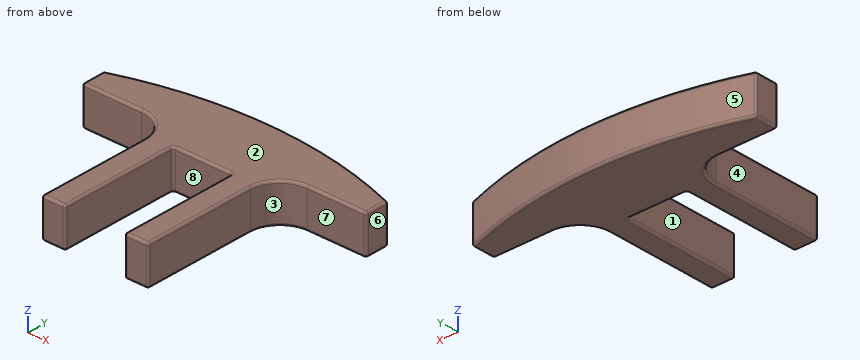
```python
from build123d import *

# Parameters (mm, degrees)
F1_DEPTH = 8.382
F2_R     = 0.508


with BuildPart() as f1:
    # F0 (on Top) → F1 (new body)
    with BuildSketch(Plane.XY):
        with BuildLine():
            Line((-16.819511, 28.70391), (-16.819511, 4.57391))
            Line((-16.819511, 4.57391), (-11.739511, 4.57391))
            Line((-11.739511, 4.57391), (-11.739511, 29.97391))
            Line((-11.739511, 29.97391), (0.960489, 29.97391))
            Line((0.960489, 29.97391), (0.960489, 4.57391))
            Line((0.960489, 4.57391), (6.040489, 4.57391))
            Line((6.040489, 4.57391), (6.040489, 28.70391))
            ThreePointArc((6.040489, 28.70391), (7.900361, 33.194038), (12.390489, 35.05391))
            Line((12.390489, 35.05391), (25.090489, 35.05391))
            Line((25.090489, 35.05391), (25.090489, 40.13391))
            ThreePointArc((25.090489, 40.13391), (-5.389511, 45.511487), (-35.869511, 40.13391))
            Line((-35.869511, 40.13391), (-35.869511, 35.05391))
            Line((-35.869511, 35.05391), (-23.169511, 35.05391))
            ThreePointArc((-23.169511, 35.05391), (-18.679383, 33.194038), (-16.819511, 28.70391))
        make_face()
    extrude(amount=F1_DEPTH)

    # F2
    f2_edges = [f1.edges().sort_by_distance(p)[0] for p in [
        (6.040489, 16.63891, 8.382),
        (3.500489, 4.57391, 8.382),
        (-35.869511, 37.59391, 8.382),
        (-29.519511, 35.05391, 8.382),
        (-18.679383, 33.194038, 8.382),
        (-16.819511, 16.63891, 8.382),
        (-14.279511, 4.57391, 8.382),
        (-11.739511, 17.27391, 8.382),
        (-5.389511, 29.97391, 8.382),
        (0.960489, 17.27391, 8.382),
        (7.900361, 33.194038, 8.382),
        (18.740489, 35.05391, 8.382),
        (25.090489, 37.59391, 8.382),
        (-5.389511, 45.511487, 8.382),
        (-5.389511, 45.511487, 0),
        (25.090489, 37.59391, 0),
        (18.740489, 35.05391, 0),
        (-35.869511, 37.59391, 0),
        (-29.519511, 35.05391, 0),
        (-18.679383, 33.194038, 0),
        (-16.819511, 16.63891, 0),
        (-14.279511, 4.57391, 0),
        (-11.739511, 17.27391, 0),
        (-5.389511, 29.97391, 0),
        (0.960489, 17.27391, 0),
        (3.500489, 4.57391, 0),
        (6.040489, 16.63891, 0),
        (7.900361, 33.194038, 0),
        (25.090489, 40.13391, 4.191),
        (-35.869511, 40.13391, 4.191),
        (12.390489, 35.05391, 4.191),
        (25.090489, 35.05391, 4.191),
        (6.040489, 4.57391, 4.191),
        (6.040489, 28.70391, 4.191),
        (0.960489, 29.97391, 4.191),
        (0.960489, 4.57391, 4.191),
        (-11.739511, 4.57391, 4.191),
        (-11.739511, 29.97391, 4.191),
        (-16.819511, 4.57391, 4.191),
        (-16.819511, 28.70391, 4.191),
        (-35.869511, 35.05391, 4.191),
        (-23.169511, 35.05391, 4.191),
    ]]
    fillet(f2_edges, radius=F2_R)


solid = f1.part
```
Check sheet for the modelled part. Datum: model origin and axes. Units: mm. Face numbers are marked on the shaded views. A direction names the side the tool comes from. Give positions to 0.01 mm unless a question says otherwise; leave off trailing zeros. Write each loop counter-clockwise with the first axis right and the second up, starting at its lowest first coordinate (ties: lowest second). Pieces come first, ordered by that corner, then holes. Notation, with made-up numbers: (10, -19) -> (21, -19) arc R9 cw to (21, -4) -> close; hole circle Ø10 at (76, 75). An arc over 180 degrees is marked (long way). Use CSV: the item, a comma, the result in double quotes. Start each with the question number.
Q1. Depth check by flat-ended pin: P1, Ø2, axis at y = 12.5, z = 2.5, coming from the -X side; P2, Ø2, axis at x = 18.5, z = 5, coming from the -Y side; P3, Ø3, axis at x = -7, z = 7, coming from the -Y side. Enter the tip coordinate at first touch or a pass-through.
Q2. Release check for a two-part mould opening along X. For the marked faces 1, 2 and 3 record: +X half, -X half, draft (parallel to the pull), parting line (faces both ways), or undercut.
Q3. Tool access check on the marked faces 4, 5, 6, 7 and 8. Record the directions out of +Z, -Z, +X, -X, +Y, -Y that give a thin tool (end or side, any length) a straight path to the whole face; none if there is none.
Q4. Scan lines: line 1 along X through (y, z) = (7.5, 4.25); line 2 along X through (y, z) = (10, 8); line 3 along Y through (x, z) = (-12.5, 6.75). Record each from-to range of solid material in increasing order.
Q5. Cross-section at B-B on z = 2.25. Enter the section's corners in (x, y), and give its area (3 significant figures).
Q6. Cross-section at A-A on y = 10. Enter the section's corners in (x, z).
Working result:
1,P1,"stops at x = -16.82"
1,P2,"stops at y = 35.05"
1,P3,"stops at y = 29.97"
2,face 1,"undercut"
2,face 2,"draft"
2,face 3,"+X half"
3,face 4,"+Z, -Z, -X, -Y"
3,face 5,"+Z, -Z, +Y"
3,face 6,"+Z, -Z, +X, +Y, -Y"
3,face 7,"+Z, -Z, +X, -Y"
3,face 8,"+Z, -Z, -Y"
4,line 1,"x = -16.82 to -11.74, 0.96 to 6.04"
4,line 2,"x = -16.8 to -11.76, 0.98 to 6.02"
4,line 3,"y = 4.57 to 45.23"
5,outline,"(-35.87, 35.56) arc R0.51 ccw to (-35.36, 35.05) -> (-23.17, 35.05) arc R6.35 cw to (-16.82, 28.7) -> (-16.82, 5.08) arc R0.51 ccw to (-16.31, 4.57) -> (-12.25, 4.57) arc R0.51 ccw to (-11.74, 5.08) -> (-11.74, 29.47) arc R0.51 cw to (-11.23, 29.97) -> (0.45, 29.97) arc R0.51 cw to (0.96, 29.47) -> (0.96, 5.08) arc R0.51 ccw to (1.47, 4.57) -> (5.53, 4.57) arc R0.51 ccw to (6.04, 5.08) -> (6.04, 28.7) arc R6.35 cw to (12.39, 35.05) -> (24.58, 35.05) arc R0.51 ccw to (25.09, 35.56) -> (25.09, 39.78) arc R0.51 ccw to (24.75, 40.26) arc R89.07 ccw to (-35.53, 40.26) arc R0.51 ccw to (-35.87, 39.78) -> close"
5,area,"921 mm^2"
6,outline,"(-16.82, 0.51) arc R0.51 ccw to (-16.31, 0) -> (-12.25, 0) arc R0.51 ccw to (-11.74, 0.51) -> (-11.74, 7.87) arc R0.51 ccw to (-12.25, 8.38) -> (-16.31, 8.38) arc R0.51 ccw to (-16.82, 7.87) -> close; (0.96, 0.51) arc R0.51 ccw to (1.47, 0) -> (5.53, 0) arc R0.51 ccw to (6.04, 0.51) -> (6.04, 7.87) arc R0.51 ccw to (5.53, 8.38) -> (1.47, 8.38) arc R0.51 ccw to (0.96, 7.87) -> close"
